Autodesk Inventor part; units mm, degrees
ref_plane "YZ Plane" through (0, 0, 0) normal (1, 0, 0) x (0, 1, 0)
ref_plane "XZ Plane" through (0, 0, 0) normal (0, 1, 0) x (-1, 0, 0)
ref_plane "XY Plane" through (0, 0, 0) normal (0, 0, 1) x (1, 0, 0)
sketch "Sketch1" plane through (0, 0, 0) normal (0, 0, 1) x (1, 0, 0)
  circle A0 centre (0, 0) radius 11
  circle A1 centre (0, 0) radius 1.75
  circle A2 centre (-8, 0) radius 1.75
  circle A3 centre (0, 8) radius 1.75
  circle A4 centre (8, 0) radius 1.75
  circle A5 centre (0, -8) radius 1.75
extrude "Extrusion1" add sketch "Sketch1" along normal blind 9.525
sketch "Sketch2" plane through (0, 0, 9.525) normal (0, 0, 1) x (1, 0, 0)
  circle A0 centre (0, 0) radius 11
  line L0 (9.0377, 6.2705) -> (14.8574, 6.2705)
  line L1 (14.8574, 6.2705) -> (14.8574, 19.7717)
  line L2 (22.8575, 28.6861) -> (24.5877, 28.6861)
  line L3 (24.5877, 28.6861) -> (24.5877, -7.2164)
  line L4 (24.5877, -7.2164) -> (8.302, -7.2164)
  line L5 (22.8575, 28.6861) -> (14.8574, 28.6861)
  line L6 (14.8574, 19.7717) -> (14.8574, 28.6861)
  point P0 (-11, -11)
extrude "Extrusion2" add sketch "Sketch2" along normal blind 23.8125
sketch "Sketch3" plane through (0, 0, 33.3375) normal (0, 0, 1) x (1, 0, 0)
  circle A0 centre (0, 0) radius 3.9688
  dimension "d4" = 7.9375
extrude "Extrusion3" cut sketch "Sketch3" against normal blind 12.4
sketch "Sketch4" plane through (0, 0, 33.3375) normal (0, 0, 1) x (1, 0, 0)
  circle A0 centre (0, 0) radius 5.5
  dimension "d7" = 11
extrude "Extrusion4" cut sketch "Sketch4" against normal blind 1.5
properties part number "goal holder flipped"
Part model, mm, in its own coordinate system. A direction names the side the tool comes from. Round coordinates to 2 decimals unless told otherwise and drop trailing zeros. Write each loop counter-clockwise with the first axis right and the second up, starting at its lowest first coordinate (ties: lowest second). Pieces come first, ordered by that corner, then holes. Notation, with made-up numbers: (-35.75, 74) -> (-16.75, 74) arc R22 ccw to (-16.75, 113) -> close; hole circle Ø6 at (1.5, -36.5). An arc over 180 degrees is marked (long way). Return JSON: item names as keys, results as strings. Group by question number.
Q1. Saw through at A-A on z = 8. Write the cut outline in (x, y).
Q2. Probe L1, parallel to Y at x = 0, z = 7; L2, parallel to X at y = 0.5, z = 5.5; L3, parallel to X at y = 27, z = 21.5. List the from-to ranges inside material, lowest first. Write a range as [from, to].
Q3. Pin check, flat tips, straight feed: pin 1 (4 mm diameter, centred on x = 16.5, y = 9.5, fed in from -Z) (3 decimals); pin 2 (6 mm diameter, centred on x = 3, z = 9, fed in from +Y); pin 3 (2 mm diameter, centred on x = 0.5, y = 2.5, fed in from +Z). Stop position of each tip, or through.
Q4. Which spindle directions (+Z, -Z, +X, -X, +Y, -Y) get a long thin tool onto all of the face, cutting with end or side? Do faces 1 (the flat face through (0, 0, 9.525)), 2 (the flat face through (12, 6.27, 21)), 3 (the cylindrical face through (-1.19, -5.37, 32.6)), 4 (the flat face through (10, 5, 33.338)). Say none if no direction does.
Q5. Saw through at D-D on z = 24. Write the cut outline in (x, y).
Q6. Mould opens along Y. For faces 5 (the flat face through (-8, 0, 9.525)), 6 (the flat face through (14.857, 17, 21)), 7 (the cylindrical face through (9.669, -0.526, 4.696)), 8 (the flat face through (17, -7.216, 21)) say: pulls with the +Y half, pulls with the -Y half, needs draft (parallel to the pull), parting line crosses it, or undercut.
Answer:
{
 "1": {"outline": "circle Ø22 at (0, 0); hole circle Ø3.5 at (-8, 0); hole circle Ø3.5 at (0, -8); hole circle Ø3.5 at (0, 0); hole circle Ø3.5 at (0, 8); hole circle Ø3.5 at (8, 0)"},
 "2": {"L1": "[-11, -9.75], [-6.25, -1.75], [1.75, 6.25], [9.75, 11]", "L2": "[-10.99, -9.68], [-6.32, -1.68], [1.68, 6.32], [9.68, 10.99]", "L3": "[14.86, 24.59]"},
 "3": {"pin 1": "z = 9.525", "pin 2": "y = 11", "pin 3": "z = 20.94"},
 "4": {"face 1": "-Z", "face 2": "+Z, -Z, +Y", "face 3": "+Z", "face 4": "+Z, +X, -X, +Y, -Y"},
 "5": {"outline": "(8.3, -7.22) -> (24.59, -7.22) -> (24.59, 28.69) -> (14.86, 28.69) -> (14.86, 6.27) -> (9.04, 6.27) arc R11 ccw (long way) to start; hole circle Ø7.94 at (0, 0)"},
 "6": {"face 5": "undercut", "face 6": "needs draft", "face 7": "undercut", "face 8": "pulls with the -Y half"}
}
